The model under review builds one solid part; all positions refer to its coordinate system, in mm. A direction names the side the tool comes from. Round coordinates to 2 decimals unless told otherwise and drop trailing zeros. Write each loop counter-clockwise with the first axis right and the second up, starting at its lowest first coordinate (ties: lowest second). Pieces come first, ordered by that corner, then holes. Notation, with made-up numbers: (35, 23) - (89, 23) arc R3 ccw to (89, 28) - close; hole circle Ø6 at (-27, 75). An arc over 180 degrees is marked (long way). Use one line per item in the form item = value.
from build123d import *

# Parameters (mm, degrees)
F0_R         = 2.05
F1_DEPTH     = 0.8
F2_DEPTH     = 19.2
F3_R         = 4.55
F4_DEPTH     = 2.1
F5_DEPTH     = 4
F6_DEPTH     = 10.3
F8_W         = 14.5
F8_H         = 16.5
F12_DEPTH    = 13.55
F13_DEPTH    = 0.65
F14_T2_ANGLE = 246.3939611614
F14_T4_ANGLE = 31.9483260065
F14_T6_ANGLE = 44.2717080563
F14_T8_ANGLE = 37.3860047758
F15_SIZE     = 0.2


# Not quite as in the source:
# - a fillet or chamfer that OpenCascade refuses, or shapes differently, is made with other operations: its cross-section is extruded or revolved along the edge and cut away or added


with BuildPart() as f1:
    # F0 (on Top) → F1 (new body)
    with BuildSketch(Plane.XY):
        with BuildLine():
            ThreePointArc((-13.5296202829, -3.5), (-13.975, 0), (-13.5296202829, 3.5))
            Line((-13.5296202829, 3.5), (-17.45, 3.5))
            ThreePointArc((-17.45, 3.5), (-20.95, 0), (-17.45, -3.5))
            Line((-17.45, -3.5), (-13.5296202829, -3.5))
        make_face()
        with Locations((-17.45, 0)):
            Circle(F0_R, mode=Mode.SUBTRACT)
    extrude(amount=F1_DEPTH)



with BuildPart() as f1b:
    # F0 (on Top) → F1, piece 2 (new body)
    with BuildSketch(Plane.XY):
        with BuildLine():
            Line((17.45, 3.5), (13.5296202829, 3.5))
            ThreePointArc((13.5296202829, 3.5), (13.975, 0), (13.5296202829, -3.5))
            Line((13.5296202829, -3.5), (17.45, -3.5))
            ThreePointArc((17.45, -3.5), (20.95, 0), (17.45, 3.5))
        make_face()
        with Locations((17.45, 0)):
            Circle(F0_R, mode=Mode.SUBTRACT)
    extrude(amount=F1_DEPTH)


with BuildPart() as f1_1:
    add(f1.part)

    add(f1b.part)  # F2 merges F1b
    # F0 (on Top) → F2 (join)
    with BuildSketch(Plane.XY):
        with BuildLine():
            ThreePointArc((13.5296202829, -3.5), (13.975, 0), (13.5296202829, 3.5))
            ThreePointArc((13.5296202829, 3.5), (0, 13.975), (-13.5296202829, 3.5))
            ThreePointArc((-13.5296202829, 3.5), (-13.975, 0), (-13.5296202829, -3.5))
            ThreePointArc((-13.5296202829, -3.5), (0, -13.975), (13.5296202829, -3.5))
        make_face()
    extrude(amount=F2_DEPTH)

    # F3 (on Top) → F4 (join)
    with BuildSketch(Plane.XY):
        with Locations((0, -7.825)):
            Circle(F3_R)
        with BuildLine():
            ThreePointArc((1.475, -5.8687599841), (2.1927437151, -6.7321253503), (2.45, -7.825))
            ThreePointArc((2.45, -7.825), (2.1927437151, -8.9178746497), (1.475, -9.7812400159))
            ThreePointArc((1.475, -9.7812400159), (0, -10.275), (-1.475, -9.7812400159))
            ThreePointArc((-1.475, -9.7812400159), (-2.45, -7.825), (-1.475, -5.8687599841))
            ThreePointArc((-1.475, -5.8687599841), (0, -5.375), (1.475, -5.8687599841))
        make_face(mode=Mode.SUBTRACT)
    extrude(amount=-F4_DEPTH)

    # F3 (on Top) → F5 (join)
    with BuildSketch(Plane.XY):
        with BuildLine():
            ThreePointArc((1.475, -9.7812400159), (2.1927437151, -8.9178746497), (2.45, -7.825))
            ThreePointArc((2.45, -7.825), (2.1927437151, -6.7321253503), (1.475, -5.8687599841))
            Line((1.475, -5.8687599841), (1.475, -9.7812400159))
        make_face()
        with BuildLine():
            Line((1.475, -9.7812400159), (1.475, -5.8687599841))
            ThreePointArc((1.475, -5.8687599841), (0, -5.375), (-1.475, -5.8687599841))
            Line((-1.475, -5.8687599841), (-1.475, -9.7812400159))
            ThreePointArc((-1.475, -9.7812400159), (0, -10.275), (1.475, -9.7812400159))
        make_face()
        with BuildLine():
            Line((-1.475, -9.7812400159), (-1.475, -5.8687599841))
            ThreePointArc((-1.475, -5.8687599841), (-2.45, -7.825), (-1.475, -9.7812400159))
        make_face()
    extrude(amount=-F5_DEPTH)

    # F3 (on Top) → F6 (join)
    with BuildSketch(Plane.XY):
        with BuildLine():
            Line((1.475, -9.7812400159), (1.475, -5.8687599841))
            ThreePointArc((1.475, -5.8687599841), (0, -5.375), (-1.475, -5.8687599841))
            Line((-1.475, -5.8687599841), (-1.475, -9.7812400159))
            ThreePointArc((-1.475, -9.7812400159), (0, -10.275), (1.475, -9.7812400159))
        make_face()
    extrude(amount=-F6_DEPTH)

    # F8 (on offset) → F9 (join, up to the next surface of F1)
    with BuildSketch(Plane.XZ.offset(-17.175)):
        with Locations((0, 8.25)):
            Rectangle(F8_W, F8_H)
    extrude(until=Until.NEXT)

    # F11 (on offset) → F12 (join)
    with BuildSketch(Plane.XY.offset(17.15)):
        with BuildLine():
            Line((-8.625, 12.9959083299), (-8.625, 11.5))
            ThreePointArc((-8.625, 11.5), (-7.9506110955, 11.9761599943), (-7.25, 12.4128209928))
            Line((-7.25, 12.4128209928), (-7.25, 13.8205759578))
            ThreePointArc((-7.25, 13.8205759578), (-7.9482026537, 13.4260870893), (-8.625, 12.9959083299))
        make_face()
        with BuildLine():
            ThreePointArc((7.25, 12.4128209928), (7.9506110955, 11.9761599943), (8.625, 11.5))
            Line((8.625, 11.5), (8.625, 12.9959083299))
            ThreePointArc((8.625, 12.9959083299), (7.9482026537, 13.4260870893), (7.25, 13.8205759578))
            Line((7.25, 13.8205759578), (7.25, 12.4128209928))
        make_face()
        with BuildLine():
            Line((8.625, 10.9959083299), (8.625, 11.5))
            ThreePointArc((8.625, 11.5), (7.9506110955, 11.9761599943), (7.25, 12.4128209928))
            ThreePointArc((7.25, 12.4128209928), (4.4752329692, 13.6606337654), (1.5, 14.2965249274))
            Line((1.5, 14.2965249274), (1.5, 13.8942659036))
            ThreePointArc((1.5, 13.8942659036), (5.2658356798, 12.9449449436), (8.625, 10.9959083299))
        make_face()
        with BuildLine():
            Line((-8.625, 11.5), (-8.625, 10.9959083299))
            ThreePointArc((-8.625, 10.9959083299), (-5.2658356798, 12.9449449436), (-1.5, 13.8942659036))
            Line((-1.5, 13.8942659036), (-1.5, 14.2965249274))
            ThreePointArc((-1.5, 14.2965249274), (-4.4752329692, 13.6606337654), (-7.25, 12.4128209928))
            ThreePointArc((-7.25, 12.4128209928), (-7.9506110955, 11.9761599943), (-8.625, 11.5))
        make_face()
    extrude(amount=-F12_DEPTH)

    # F11 (on offset) → F13 (cut, through all)
    with BuildSketch(Plane.XY.offset(17.15)):
        with BuildLine():
            Line((-8.625, 12.9959083299), (-8.625, 11.5))
            ThreePointArc((-8.625, 11.5), (-7.9506110955, 11.9761599943), (-7.25, 12.4128209928))
            Line((-7.25, 12.4128209928), (-7.25, 13.8205759578))
            ThreePointArc((-7.25, 13.8205759578), (-7.9482026537, 13.4260870893), (-8.625, 12.9959083299))
        make_face()
        with BuildLine():
            ThreePointArc((7.25, 12.4128209928), (7.9506110955, 11.9761599943), (8.625, 11.5))
            Line((8.625, 11.5), (8.625, 12.9959083299))
            ThreePointArc((8.625, 12.9959083299), (7.9482026537, 13.4260870893), (7.25, 13.8205759578))
            Line((7.25, 13.8205759578), (7.25, 12.4128209928))
        make_face()
    extrude(amount=-F13_DEPTH, mode=Mode.SUBTRACT)

    # F14: fillet of radius 2.1 on 1 edges, made by hand

    # F14_s1 → F14_t2 (revolve, cut)
    with BuildSketch(Plane(origin=(0, 0, 0), x_dir=(0, 0, 1), z_dir=(-0.2504472272, 0.9681302528, 0))):
        with BuildLine():
            ThreePointArc((17.1, 13.975), (18.5849242405, 13.3599242405), (19.2, 11.875))
            Line((19.2, 11.875), (19.242, 11.875))
            Line((19.242, 11.875), (19.242, 14.017))
            Line((19.242, 14.017), (17.1, 14.017))
            Line((17.1, 14.017), (17.1, 13.975))
        make_face()
    revolve(axis=Axis((0, 0, 19.2), (0, 0, -1)), revolution_arc=F14_T2_ANGLE, mode=Mode.SUBTRACT)

    # F14_s3 → F14_t4 (revolve, cut)
    with BuildSketch(Plane(origin=(0, 0, 0), x_dir=(0, 0, 1), z_dir=(-0.7868271317, -0.617173448, 0))):
        with BuildLine():
            ThreePointArc((17.15, 13.975), (18.6024979201, 13.3427353976), (19.2, 11.8755953225))
            Line((19.2, 11.8755953225), (19.242, 11.8755953225))
            Line((19.242, 11.8755953225), (19.242, 13.975))
            Line((19.242, 13.975), (19.2, 14.017))
            ThreePointArc((19.2, 14.017), (18.175, 14.017), (17.151, 14.0169880936))
            Line((17.151, 14.0169880936), (17.15, 13.975))
        make_face()
    revolve(axis=Axis((0, 0, 19.2), (0, 0, -1)), revolution_arc=F14_T4_ANGLE, mode=Mode.SUBTRACT)

    # F14_s5 → F14_t6 (revolve, cut)
    with BuildSketch(Plane(origin=(0, 0, 0), x_dir=(0, 0, 1), z_dir=(-0.9942229517, -0.1073346275, 0))):
        with BuildLine():
            ThreePointArc((17.15, 13.975), (18.6024979201, 13.3427353976), (19.2, 11.8755953225))
            Line((19.2, 11.8755953225), (19.242, 11.8755953225))
            Line((19.242, 11.8755953225), (19.242, 13.975))
            Line((19.242, 13.975), (19.2, 14.017))
            ThreePointArc((19.2, 14.017), (18.175, 14.017), (17.151, 14.0169880936))
            Line((17.151, 14.0169880936), (17.15, 13.975))
        make_face()
    revolve(axis=Axis((0, 0, 19.2), (0, 0, -1)), revolution_arc=F14_T6_ANGLE, mode=Mode.SUBTRACT)

    # F14_s7 → F14_t8 (revolve, cut)
    with BuildSketch(Plane(origin=(0, 0, 0), x_dir=(0, 0, 1), z_dir=(-0.7868271352, 0.6171734435, 0))):
        with BuildLine():
            ThreePointArc((17.1, 13.975), (18.5849242405, 13.3599242405), (19.2, 11.875))
            Line((19.2, 11.875), (19.242, 11.875))
            Line((19.242, 11.875), (19.242, 14.017))
            Line((19.242, 14.017), (17.1, 14.017))
            Line((17.1, 14.017), (17.1, 13.975))
        make_face()
    revolve(axis=Axis((0, 0, 19.2), (0, 0, -1)), revolution_arc=F14_T8_ANGLE, mode=Mode.SUBTRACT)

    # F15
    f15_edges = [f1_1.edges().sort_by_distance(p)[0] for p in [
        (0, -5.375, -10.3),
        (0, -10.275, -10.3),
    ]]
    chamfer(f15_edges, length=F15_SIZE)


solid = f1_1.part
(1) Add section D-D on x = 18. Write out the cut boundary in (y, z), then the cut area to 3 significant figures.
Geometry results:
outline = (-3.46, 0) - (-1.97, 0) - (-1.97, 0.8) - (-3.46, 0.8) - close; (1.97, 0) - (3.46, 0) - (3.46, 0.8) - (1.97, 0.8) - close
area = 2.37 mm2
(2) Add section C-C on z = 2. Write out the cut boundary in (x, y) (3 decimals), then the cut area to 3 significant figures.
Geometry results:
outline = (-7.25, 11.947) arc R13.975 ccw (long way) to (7.25, 11.947) - (7.25, 17.175) - (-7.25, 17.175) - close
area = 669 mm2
(3) To check wall thickness, follow L1, parallel to Y at x = -17.45, z = 0.45; L2, parallel to Z at x = -14.5, y = 1.5; L3, parallel to Z at x = -3, y = 2. State the ranges of each line that lie inside material, in increasing order.
Geometry results:
L1 = -3.5 to -2.05, 2.05 to 3.5
L2 = 0 to 0.8
L3 = 0 to 19.2
(4) The part is to be moulded in two halves that separate along Y. For faces 4 (the cylindrical face through (19.34, -0.79, 0.39)), 5 (the cylindrical face through (-19.5, 0.09, 0.39)), 6 (the flat face through (-16, -2, 0.8)), 7 (the flat face through (0, 17.175, 8)), say which applies: +Y half, -Y half, draft (parallel to the pull), parting line (faces both ways), or undercut.
Geometry results:
face_4 = undercut
face_5 = undercut
face_6 = draft
face_7 = +Y half
(5) Add section A-A on y = 0. Write out the cut boundary in (x, z) (3 decimals).
Geometry results:
outline = (-20.95, 0) - (-19.5, 0) - (-19.5, 0.8) - (-20.95, 0.8) - close; (-15.4, 0) - (15.4, 0) - (15.4, 0.8) - (13.975, 0.8) - (13.975, 17.1) arc R2.1 ccw to (11.875, 19.2) - (-11.875, 19.2) arc R2.1 ccw to (-13.975, 17.1) - (-13.975, 0.8) - (-15.4, 0.8) - close; (19.5, 0) - (20.95, 0) - (20.95, 0.8) - (19.5, 0.8) - close
(6) Add section B-B on x = 0. Write out the cut boundary in (y, z) (3 decimals), then the cut area to 3 significant figures.
Geometry results:
outline = (-13.975, 0) - (-12.375, 0) - (-12.375, -2.1) - (-10.275, -2.1) - (-10.275, -10.1) - (-10.075, -10.3) - (-5.575, -10.3) - (-5.375, -10.1) - (-5.375, -2.1) - (-3.275, -2.1) - (-3.275, 0) - (17.175, 0) - (17.175, 16.5) - (13.975, 16.5) - (13.975, 17.15) arc R2.1 ccw to (11.876, 19.2) - (-11.875, 19.2) arc R2.1 ccw to (-13.975, 17.1) - close
area = 647 mm2
(7) Insertion check: P1, Ø10, axis at x = -15, z = 4, coming from the -Y side; P2, Ø4, axis at y = 13.5, z = 11.5, coming from the +X side (3 decimals); P3, Ø6.5, axis at x = 17.45, y = 0, coming from the -Z side. Each pin has a flat end and moves straight along its axis. Give the tip position at first contact, or say it passes through.
Geometry results:
P1 = -9.76
P2 = 8.625
P3 = 0
(8) Machinability: for faces 1 (the flat face through (8, 12, 3.6)), 2 (the flat face through (5.3, 13.1, 17.15)), 3 (the flat face through (-2, -8, -4)), which of the approach directions +Z, -Z, +X, -X, +Y, -Y give a long, thin tool a straight path to every point of the face, cutting with its end or side? Answer none if there is none.
Geometry results:
face_1 = -Z, +X, +Y
face_2 = +Z, +X, +Y
face_3 = -Z, -X, +Y, -Y
